For this review, use the dimensioned drawing (mm, ordinates from the lowest corner) and the shaded views. A direction names the side the tool comes from. Give positions to 0.01 mm unless a question says otherwise; leave off trailing zeros. Order: outer loops, then holes, each group sorted by start corner. A loop starts at its lowest first (then second) coordinate and runs counter-clockwise, first axis right, second up.
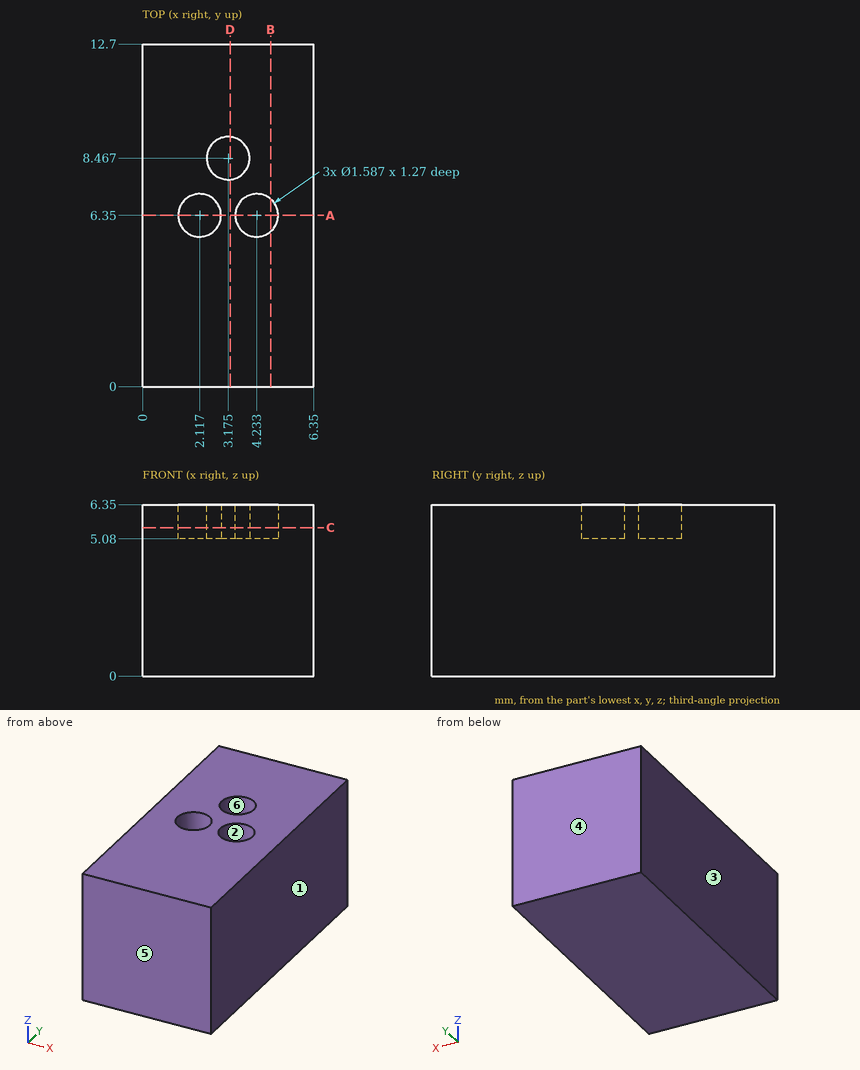
1. Take a section at C-C (z = 5.5). Count the separate pieces of the cut face and the enclosed holes in it.
2. To check wall thickness, follow line 1 (Z direction, x = 3.75, y = 8); line 2 (Y direction, x = 1.75, z = 5.5) (1 decimal). State the ranges of each line that lie inside material, in increasing order.
3. Take a section at D-D (x = 3.25). Write out the cut boundary in (y, z).
4. Insertion check: pin 1 (0.8 mm diameter, centred on x = 4.5, y = 6, fed in from +Z). The pin has a flat end and moves straight along its axis. Give the tip position at first contact, or say it passes through.
5. For the marked faces 5 and 6, list the 3-axis set-ups (+Z, -Z, +X, -X, +Y, -Y) from which the entire face can be reached by the end or side of a thin tool; tool diameter is ignored.
6. Take a section at B-B (x = 4.75). Write out the cut boundary in (y, z).
7. Draft analysis for pull direction X (two halves, no side actions). For the marked faces 1, 2, 3 and 4, state which applies: pulls with the +X half, pulls with the -X half, needs draft (parallel to the pull), parting line crosses it, or undercut.
8. Take a section at A-A (y = 6.35). Write out the cut boundary in (x, z).
Answer:
1. separate pieces: 1
1. enclosed holes: 3
2. line 1: z = 0 to 5.08
2. line 2: y = 0 to 5.6, 7.1 to 12.7
3. outline: (0, 0) - (12.7, 0) - (12.7, 6.35) - (9.26, 6.35) - (9.26, 5.08) - (7.68, 5.08) - (7.68, 6.35) - (0, 6.35) - close
4. pin 1: stops at z = 6.35
5. face 5: +Z, -Z, +X, -X, -Y
5. face 6: +Z
6. outline: (0, 0) - (12.7, 0) - (12.7, 6.35) - (6.95, 6.35) - (6.95, 5.08) - (5.75, 5.08) - (5.75, 6.35) - (0, 6.35) - close
7. face 1: pulls with the +X half
7. face 2: undercut
7. face 3: pulls with the -X half
7. face 4: needs draft
8. outline: (0, 0) - (6.35, 0) - (6.35, 6.35) - (5.03, 6.35) - (5.03, 5.08) - (3.44, 5.08) - (3.44, 6.35) - (2.91, 6.35) - (2.91, 5.08) - (1.32, 5.08) - (1.32, 6.35) - (0, 6.35) - close
